Part model, mm, in its own coordinate system. A direction names the side the tool comes from. Give positions to 0.01 mm unless a question says otherwise; leave off trailing zeros. Write each loop counter-clockwise with the first axis right and the second up, starting at its lowest first coordinate (ties: lowest second). Pieces come first, ordered by that corner, then holes.
from build123d import *

# Parameters (mm, degrees)
BASE_EXTRUDE_DEPTH = 20
CUT_EXTRUDE2_DEPTH = 233.044057119


with BuildPart() as part:
    # Sketch1 → Base-Extrude (new body)
    with BuildSketch(Plane.XY):
        with BuildLine():
            Line((-90, -100), (110, -100))
            Line((110, -100), (110, 100))
            ThreePointArc((110, 100), (104.72135955, 122.360679775), (90, 140))
            Line((90, 140), (-30, 200))
            ThreePointArc((-30, 200), (-70.70367517, 196.055512755), (-90, 160))
            Line((-90, 160), (-90, -100))
        make_face()
    extrude(amount=BASE_EXTRUDE_DEPTH)

    # Sketch3 → Cut-Extrude2 (cut, through all)
    with BuildSketch(Plane(origin=(0, 0, 0), x_dir=(-1, 0, 0), z_dir=(0, 0, -1))):
        with BuildLine():
            Line((2.736269939, 124.876265588), (-41.180339887, 102.917960675))
            ThreePointArc((-41.180339887, 102.917960675), (-51.266270209, 93.700558703), (-55, 80.5572809))
            Line((-55, 80.5572809), (-55, -35))
            ThreePointArc((-55, -35), (-52.071067812, -42.071067812), (-45, -45))
            Line((-45, -45), (25, -45))
            ThreePointArc((25, -45), (32.071067812, -42.071067812), (35, -35))
            Line((35, -35), (35, 104.968443396))
            ThreePointArc((35, 104.968443396), (34.015369025, 107.947841254), (31.449275362, 109.753796144))
            ThreePointArc((31.449275362, 109.753796144), (19.107472836, 115.315093875), (8.597931721, 123.847248796))
            ThreePointArc((8.597931721, 123.847248796), (5.836869232, 125.328821056), (2.736269939, 124.876265588))
        make_face()
    extrude(amount=-CUT_EXTRUDE2_DEPTH, mode=Mode.SUBTRACT)


solid = part.part
1) Mould opens along Y. For faces 3 (the cylindrical face through (52.15, -41.99, 9.86)), 4 (the flat face through (30.8, 169.6, 9.9)), 5 (the flat face through (-36, 54, 20)), 6 (the flat face through (55, 24, 10)) say: +Y half, -Y half, draft (parallel to the pull), parting line (faces both ways), or undercut.
Check result:
face 3: undercut
face 4: +Y half
face 5: draft
face 6: undercut
2) Drill centre lines: L1, parallel to X at y = 22, z = 5; L2, parallel to Y at x = -21, z = 15.75; L3, parallel to Y at x = 41, z = 12.25. Where is each one in solid material? Low to high.
Check result:
L1: x = -90 to -35, 55 to 110
L2: y = -100 to -45, 114.2 to 195.5
L3: y = -100 to -45, 103.01 to 164.5
3) Saw through at C-C (x = 83). Write the cut outline in (y, z).
Check result:
outline: (-100, 0) - (143.5, 0) - (143.5, 20) - (-100, 20) - close
4) Flat gauge pins, fed straight in: P1, Ø5, axis at y = 165, z = 7, coming from the -X side; P2, Ø4, axis at x = 51.5, z = 12.5, coming from the +Y side; P3, Ø1, axis at x = 30.5, z = 14, coming from the +Y side. Where does each tip first touch, or does it go through?
Check result:
P1: stops at x = -89.93
P2: stops at y = 160.25
P3: stops at y = 170
5) Saw through at B-B (x = 17.5). Write the cut outline in (y, z), and give its area (3 significant figures).
Check result:
outline: (-100, 0) - (-45, 0) - (-45, 20) - (-100, 20) - close; (114.76, 0) - (176.25, 0) - (176.25, 20) - (114.76, 20) - close
area: 2,330 mm2
6) Saw through at A-A (z = 15.25). Write the cut outline in (x, y).
Check result:
outline: (-90, -100) - (110, -100) - (110, 100) arc R50 ccw to (90, 140) - (-30, 200) arc R43.33 ccw to (-90, 160) - close; hole (-35, -35) arc R10 ccw to (-25, -45) - (45, -45) arc R10 ccw to (55, -35) - (55, 80.56) arc R25 ccw to (41.18, 102.92) - (-2.74, 124.88) arc R5 ccw to (-8.6, 123.85) arc R52.5 cw to (-31.45, 109.75) arc R5 ccw to (-35, 104.97) - close
7) Saw through at D-D (y = 170). Write the cut outline in (x, z).
Check result:
outline: (-88.83, 0) - (30, 0) - (30, 20) - (-88.83, 20) - close
8) 3-axis set-ups, long thin cutter, end or side, ignore diameter. For faces 1 (the cylindrical face through (-5.88, 125.32, 9.86)), 2 (the flat face through (-90, 32, 10)): which of +Z, -Z, +X, -X, +Y, -Y reach the whole face in a straight line?
Check result:
face 1: +Z, -Z
face 2: +Z, -Z, -X, +Y, -Y
